Answer from the drawing. Dimensions are ordinates in mm from the lowest x, y and z of the part. Coordinates: 2 decimals unless noted, no trailing zeros. Order: outer loops, then holes, each group sorted by start corner. A loop starts at its lowest first (then second) coordinate and runs counter-clockwise, first axis right, second up. Notation, with made-up numbers: M 36,21.5 L 66,21.5 A5 ccw 66,28.5 Z; hole C -6.5,43.5 d11. An arc over 180 degrees is marked long. Write each question's results on one line, items separated by ' | '.
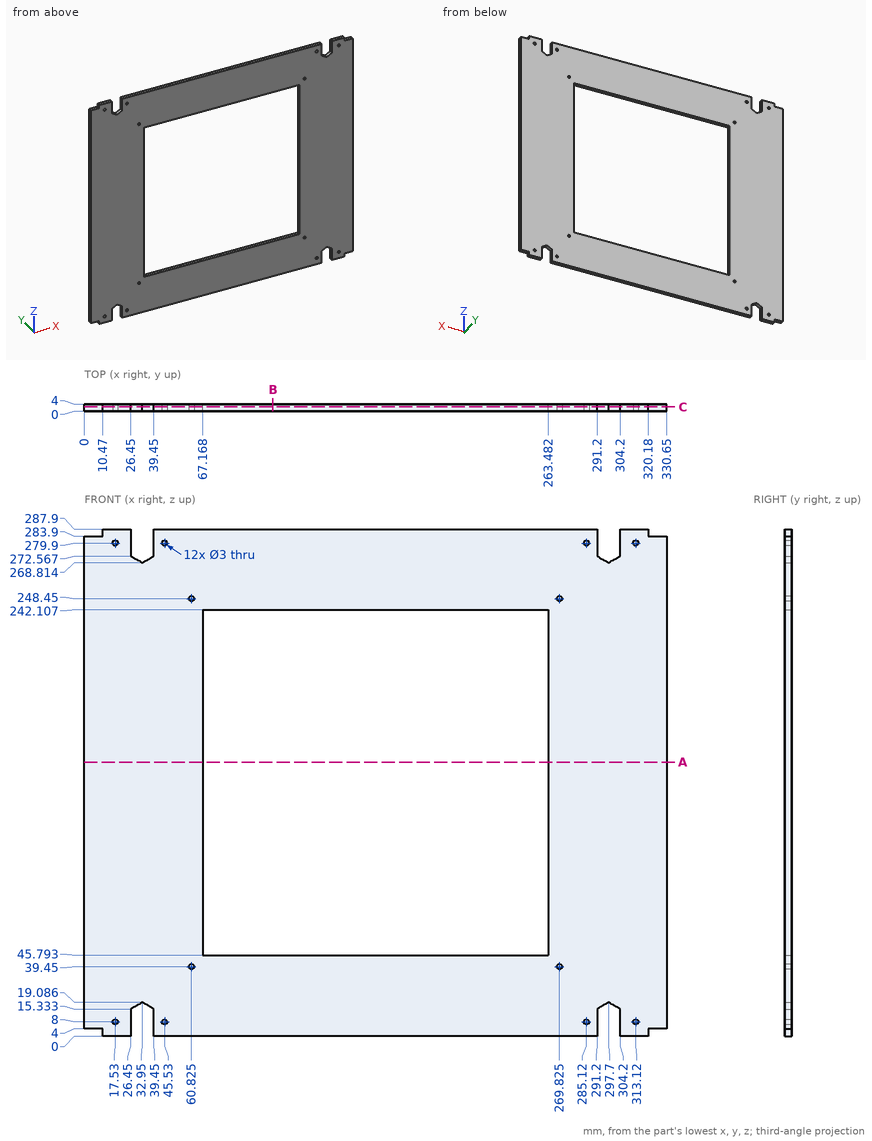
(1) The part is cut by section C-C, the plane y = 2.3. Count the separate pieces of the cut face and the enclosed holes in it, then the cut area to 3 significant figures.
Conclusion:
separate pieces: 1 | enclosed holes: 13 | area: 55,500 mm²
(2) The part is cut by section B-B, the plane x = 107. Write down the section's boundary in (y, z).
Conclusion:
outline: M 0,0 L 4,0 L 4,45.79 L 0,45.79 Z; M 0,242.11 L 4,242.11 L 4,287.9 L 0,287.9 Z
(3) The part is cut by section A-A, the plane z = 155.5. Write down the section's boundary in (x, y).
Conclusion:
outline: M 0,0 L 67.17,0 L 67.17,4 L 0,4 Z; M 263.48,0 L 330.65,0 L 330.65,4 L 263.48,4 Z
(4) Straight lines are drawn through the part: line 1 (Z direction, x = 285.12, y = 1.7); line 2 (X direction, y = 1.75, z = 62.5); line 3 (Z direction, x = 239.5, y = 3.05). For each, find the intervals that lie inside material, in ascending order.
Conclusion:
line 1: 0 to 6.5, 9.5 to 278.4, 281.4 to 287.9 | line 2: 0 to 67.17, 263.48 to 330.65 | line 3: 0 to 45.79, 242.11 to 287.9
